from build123d import *

# Parameters (mm, degrees)
SKETCH_1_R          = 2.5
EXTRUDE_1_DEPTH     = 10
SKETCH_2_R          = 2
CUT_EXTRUDE_2_DEPTH = 18.18324903


with BuildPart() as part:
    # Эскиз1 → Вытянуть1 (new body)
    with BuildSketch(Plane.XY):
        Polygon((3.560836522, 4), (4.560836522, 3), (4.560836522, -3), (3.560836522, -4), (-13.388952432, -4), (-13.388952432, 0), (-5.665361164, 0), (-5.665361164, 4), align=None)
        Circle(SKETCH_1_R, mode=Mode.SUBTRACT)
    extrude(amount=EXTRUDE_1_DEPTH)

    # Эскиз2 → Вытянуть2 (cut, through all)
    with BuildSketch(Plane(origin=(0, 0, 0), x_dir=(-1, 0, 0), z_dir=(0, 1, 0))):
        with Locations(Location((10.466786093, 5, 0), (0, 0, 90))):
            Circle(SKETCH_2_R)
    extrude(amount=-CUT_EXTRUDE_2_DEPTH, mode=Mode.SUBTRACT)


solid = part.part
Input: part model. Units: mm. Frame: model coordinates. A direction names the side the tool comes from. Round coordinates to 2 decimals unless told otherwise and drop trailing zeros. Order: outer loops, then holes, each group sorted by start corner. A loop starts at its lowest first (then second) coordinate and runs counter-clockwise, first axis right, second up.
1. Mould query, pull axis X, two halves, no side actions, for faces 1 (the face through (-5, -4, 5)), 2 (the face through (-13.389, -2, 5)), 3 (the face through (-11.68, -1.97, 3.41)). Classes: released by +X, released by -X, zero draft, split by the parting line, or undercut.
The answers:
face 1: zero draft
face 2: released by -X
face 3: undercut
2. Cut plane A-A, the plane z = 5. Output: boundary loops of the cut face in (x, y).
The answers:
outline: (-13.39, -4) - (-12.47, -4) - (-12.47, 0) - (-13.39, 0) - close; (-8.47, -4) - (3.56, -4) - (4.56, -3) - (4.56, 3) - (3.56, 4) - (-5.67, 4) - (-5.67, 0) - (-8.47, 0) - close; hole circle Ø5 at (0, 0)
3. Set-up query: faces 4 (the face through (4.07, -3.49, 4.93)), 5 (the face through (-5.665, 2, 5)). Return all of +Z, -Z, +X, -X, +Y, -Y with unobstructed straight access to the full face (end or side cutting, diameter ignored); none if empty.
The answers:
face 4: +Z, -Z, +X, -Y
face 5: +Z, -Z, -X, +Y
4. Cut plane D-D, the plane z = 8.5. Output: boundary loops of the cut face in (x, y), then the cut area to 3 significant figures.
The answers:
outline: (-13.39, -4) - (3.56, -4) - (4.56, -3) - (4.56, 3) - (3.56, 4) - (-5.67, 4) - (-5.67, 0) - (-13.39, 0) - close; hole circle Ø5 at (0, 0)
area: 92.1 mm2
5. Material intervals for line 1 (Y direction, x = 0, z = 3); line 2 (X direction, y = -1.75, z = 3.5); line 3 (X direction, y = -0.75, z = 4.75), sorted ascending.
The answers:
line 1: y = -4 to -2.5, 2.5 to 4
line 2: x = -13.39 to -11.79, -9.14 to -1.79, 1.79 to 4.56
line 3: x = -13.39 to -12.45, -8.48 to -2.38, 2.38 to 4.56
6. Cut plane B-B, the plane y = 1.5. Output: boundary loops of the cut face in (x, z), then the cut area to 3 significant figures.
The answers:
outline: (-5.67, 0) - (-2, 0) - (-2, 10) - (-5.67, 10) - close; (2, 0) - (4.56, 0) - (4.56, 10) - (2, 10) - close
area: 62.3 mm2
7. Cut plane C-C, the plane x = 0. Output: boundary loops of the cut face in (y, z).
The answers:
outline: (-4, 0) - (-2.5, 0) - (-2.5, 10) - (-4, 10) - close; (2.5, 0) - (4, 0) - (4, 10) - (2.5, 10) - close
8. Pin query (flat end, axial travel): P1, Ø1, axis at x = -1, y = 1, coming from the -Z side; P2, Ø2.5, axis at x = -8, z = 4.5, coming from the +Y side. Return the tip coordinate at first contact, or that it passes through.
The answers:
P1: passes through
P2: stops at y = 0
